Can you work these out from the model? Positions are in its coordinate system, mm. A direction names the side the tool comes from. Coordinates: 2 decimals unless noted, no trailing zeros. Order: outer loops, then holes, each group sorted by start corner. A loop starts at its lowest first (then second) coordinate and runs counter-clockwise, first axis right, second up. Notation, with made-up numbers: (13, -22.5) -> (67, -22.5) arc R25 ccw to (67, -4.5) -> close; hole circle Ø10 at (22.25, 48). An arc over 180 degrees is marked (long way). Write item = value, one per line.
Autodesk Inventor part; units mm, degrees
ref_plane "YZ Plane" through (0, 0, 0) normal (1, 0, 0) x (0, 1, 0)
ref_plane "XZ Plane" through (0, 0, 0) normal (0, 1, 0) x (-1, 0, 0)
ref_plane "XY Plane" through (0, 0, 0) normal (0, 0, 1) x (1, 0, 0)
ref_plane "Płaszczyzna konstrukcyjna1" through (0, 0, 0) normal (0, 0, 1) x (1, 0, 0)
sketch "Szkic1" plane through (0, 0, 0) normal (0, 0, 1) x (1, 0, 0)
  circle A0 centre (90, 0) radius 90
  circle A1 centre (90, 0) radius 80
  circle A2 centre (90, 0) radius 80
  circle A3 centre (90, 0) radius 72.5
  circle A4 centre (90, 0) radius 30
  point P0 (0, 0)
  dimension "d0" = 145
  dimension "d1" = 60
extrude "Wyciągnięcie proste1" add sketch "Szkic1" along normal blind 5 contours A0 | A1 | A3
sketch "Szkic2" plane through (90, 0, 0) normal (0, 0, -1) x (-1, 0, 0)
  circle A0 centre (0, 0) radius 30
  circle A1 centre (0, 0) radius 32.5
  point P0 (90, 0)
  dimension "d4" = 65
extrude "Wyciągnięcie proste2" add sketch "Szkic2" along normal blind 150
sketch "Szkic3" plane through (90, 0, -150) normal (0, 0, -1) x (-1, 0, 0)
  circle A0 centre (0, 0) radius 32.5
  point P0 (90, 0)
extrude "Wyciągnięcie proste3" add sketch "Szkic3" along normal blind 3
chamfer "Faza1" distance 1 angle 45 1 edges at (122.5, 0, -153)
chamfer "Faza2" distance 5 angle 45 1 edges at (60, 0, 5)
sketch "Szkic4" plane through (90, 0, 0) normal (0, 0, -1) x (-1, 0, 0)
  circle A0 centre (0, 0) radius 80
  circle A1 centre (0, 0) radius 80
  circle A2 centre (0, 0) radius 72.5
  point P0 (90, 0)
  dimension "d15" = 145
extrude "Wyciągnięcie proste4" add sketch "Szkic4" along normal blind 10
chamfer "Faza3" distance 1 angle 45 5 edges at (0, 0, 5) (0, 0, 0) (170, 0, -10) (162.5, 0, -10) (122.5, 0, 0)
properties part number "dekiel" material "Stal nierdzewna"
Item 1: If I drill on probe 1 along Y at (x, z) = (90, -85); probe 2 along Y at (x, z) = (71.5, -4); probe 3 along Y at (x, z) = (90, 0.05), over which ranges is the centre line in solid material (lowest first)?
A:
probe_1 = -32.5 to -30, 30 to 32.5
probe_2 = -77.83 to -70.1, -26.72 to -23.62, 23.62 to 26.72, 70.1 to 77.83
probe_3 = -89.05 to -30.05, 30.05 to 89.05
Item 2: For faces 5 (the flat face through (90, 0, -150)), 6 (the flat face through (20, -23, -10)), 7 (the cylindrical face through (18.579, 54.764, 2.479)), which set-ups out of +Z, -Z, +X, -X, +Y, -Y let a thin tool reach every point of the face, with its end or its side?
A:
face_5 = +Z
face_6 = -Z
face_7 = +Z, -Z
Item 3: If we mould it in two halves opening along X, with no side actions, what happens to faces 1 (the cylindrical face through (162.43, -3.19, -4.44)), 2 (the flat face through (105, -31, 0)), 3 (the cylindrical face through (13.694, -24.03, -4.437)), 4 (the flat face through (89, -38, 5))? For each: pulls with the +X half, pulls with the -X half, needs draft (parallel to the pull), parting line crosses it, or undercut.
A:
face_1 = undercut
face_2 = undercut
face_3 = parting line crosses it
face_4 = needs draft
Item 4: I'm going to push flat-ended pins straight in: P1, Ø5, axis at x = 114, y = -40, coming from the -Z side; P2, Ø8, axis at x = 80.5, y = -3, coming from the +Z side; P3, Ø8, axis at y = -9, z = -113, coming from the -X side. Where does each tip first touch, or does it pass through?
A:
P1 = 0
P2 = -150
P3 = 57.89
Item 5: I want a section at C-C, the plane z = -57.5. Please give me the cut outline in (x, y).
A:
outline = circle Ø65 at (90, 0); hole circle Ø60 at (90, 0)
